Check sheet for the modelled part. Datum: model origin and axes. Units: mm. A direction names the side the tool comes from. Give positions to 0.01 mm unless a question says otherwise; leave off trailing zeros. Order: outer loops, then holes, each group sorted by start corner. A loop starts at its lowest first (then second) coordinate and runs counter-clockwise, first axis right, second up. Notation, with made-up numbers: M 52,67.5 L 72,67.5 A19 ccw 72,80.5 Z; hole C 9.5,22.5 d2. An arc over 180 degrees is marked long. Answer in a Markdown table with one row per item. Add a question column.
from build123d import *

# Parameters (mm, degrees)
SKETCH1_R           = 1.6500000000000001
SKETCH1_R_2         = 1.6500000000000006
BOSS_EXTRUDE1_DEPTH = 2
BOSS_EXTRUDE2_DEPTH = 2
BOSS_EXTRUDE3_DEPTH = 4
SKETCH4_R           = 1.8999999999999948
SKETCH4_R_2         = 1.8999999999999981
CUT_EXTRUDE1_DEPTH  = 4
SKETCH5_R           = 1.0000000000000009
SKETCH5_R_2         = 1
SKETCH5_R_3         = 1.8999999999999981
CUT_EXTRUDE2_DEPTH  = 63.418667079648536
CUT_EXTRUDE3_DEPTH  = 4
CHAMFER1_SIZE       = 5
CHAMFER2_SIZE       = 2
FILLET1_R           = 8
FILLET2_R           = 8
FILLET3_R           = 8


# Some blends are built 0.0001 mm under size
with BuildPart() as part:
    # Sketch1 → Boss-Extrude1 (new body)
    with BuildSketch(Plane.XY):
        Polygon((0, 0), (-12, -1.47e-15), (-12, 45), (0, 45), align=None)
        with Locations((-6.499999999999999, 37)):
            Circle(SKETCH1_R, mode=Mode.SUBTRACT)
        with Locations((-6.5000000000000036, 5.999999999999999)):
            Circle(SKETCH1_R_2, mode=Mode.SUBTRACT)
    extrude(amount=-BOSS_EXTRUDE1_DEPTH)

    # Sketch2 → Boss-Extrude2 (add)
    with BuildSketch(Plane(origin=(0, 0, 0), x_dir=(0, 0, -1), z_dir=(1, 0, 0))):
        Polygon((35.3, 45), (2, 0), (5.51e-15, 0), (0, 45), align=None)
    extrude(amount=BOSS_EXTRUDE2_DEPTH)

    # Sketch3 → Boss-Extrude3 (add)
    with BuildSketch(Plane(origin=(0, 45, 0), x_dir=(1, 0, 0), z_dir=(0, 1, 0))):
        Polygon((-6.1e-16, 35.3), (25, 35.3), (25.000000000000004, 1.9999999999999991), (3.47e-15, 1.9999999999999991), align=None)
    extrude(amount=-BOSS_EXTRUDE3_DEPTH)

    # Sketch4 → Cut-Extrude1 (cut)
    with BuildSketch(Plane(origin=(0, 45, 0), x_dir=(1, 0, 0), z_dir=(0, 1, 0))):
        with Locations(Location((20.000000000000004, 26.850000000000005, 0), (0, 0, 270))):
            Circle(SKETCH4_R)
        with Locations(Location((20.00000000000001, 16.45, 0), (0, 0, 270))):
            Circle(SKETCH4_R)
        with Locations(Location((11.200000000000008, 21.650000000000002, 0), (0, 0, 270))):
            Circle(SKETCH4_R_2)
    extrude(amount=-CUT_EXTRUDE1_DEPTH, mode=Mode.SUBTRACT)

    # Sketch5 → Cut-Extrude2 (cut, through all)
    with BuildSketch(Plane(origin=(0, 45, 0), x_dir=(1, 0, 0), z_dir=(0, 1, 0))):
        with Locations(Location((3.5826389249908894, 23.65, 0), (0, 0, 270))):
            Circle(SKETCH5_R)
        with Locations(Location((3.5826389249908894, 19.650000000000002, 0), (0, 0, 270))):
            Circle(SKETCH5_R_2)
        with Locations(Location((11.200000000000008, 21.650000000000002, 0), (0, 0, 270))):
            Circle(SKETCH5_R_3)
    extrude(amount=-CUT_EXTRUDE2_DEPTH, mode=Mode.SUBTRACT)

    # Sketch6 → Cut-Extrude3 (cut)
    with BuildSketch(Plane(origin=(0, 45, 0), x_dir=(1, 0, 0), z_dir=(0, 1, 0))):
        Polygon((13.000000000000005, 1.9999999999999991), (25.000000000000004, 13.999999999999877), (25.000000000000004, 1.9999999999999991), align=None)
    extrude(amount=-CUT_EXTRUDE3_DEPTH, mode=Mode.SUBTRACT)

    # Chamfer1
    # the kernel refuses this chamfer: 5 mm, written as the material it adds along each edge
    with BuildSketch(Plane(origin=(2, 41, -45.19841493982955), x_dir=(-0.02749587661058636, -0.9996219169112968, 0), z_dir=(0, 0, 1))) as chamfer1_piece_1_section:
        Polygon((CHAMFER1_SIZE * 0.999621916911, CHAMFER1_SIZE * 0.0274958766106), (-CHAMFER1_SIZE * 0.0274958766106, CHAMFER1_SIZE * 0.999621916911), (0, 0), align=None)
    chamfer1_piece_1 = extrude(amount=43.19841493982955, mode=Mode.PRIVATE)
    chamfer1_piece_1 = split(chamfer1_piece_1, bisect_by=Plane(origin=(3.679771833975431, 32.284665683470884, -25.89065260576845), z_dir=(0, 0.5948430054102947, 0.8038418992031009)), keep=Keep.TOP, mode=Mode.PRIVATE)
    chamfer1_piece_1 = chamfer1_piece_1 - Plane(origin=(3.5826389249908894, 39.396771086693036, -19.650000000000002), x_dir=(-1.8e-16, 0, 1), z_dir=(0, 1, 0)) * Cylinder(1, 107, mode=Mode.PRIVATE)
    chamfer1_piece_1 = chamfer1_piece_1 - Plane(origin=(3.5826389249908894, 39.396771086693036, -23.65), x_dir=(-1.8e-16, 0, 1), z_dir=(0, 1, 0)) * Cylinder(1.0000000000000009, 107, mode=Mode.PRIVATE)
    add(chamfer1_piece_1)

    # Chamfer2
    chamfer2_edges = [part.edges().sort_by_distance(p)[0] for p in [
        (1.9999999999990004, 40.50000000000074, -1.9999999999999996),
    ]]
    chamfer(chamfer2_edges, length=CHAMFER2_SIZE - 0.0001)  # a hair under: the kernel refuses the full size

    # Fillet1
    fillet1_edges = [part.edges().sort_by_distance(p)[0] for p in [
        (-12, -1.47e-15, -1),
        (-12, 45, -1),
    ]]
    fillet(fillet1_edges, radius=FILLET1_R)

    # Fillet2
    fillet2_edges = [part.edges().sort_by_distance(p)[0] for p in [
        (-6.1e-16, 43, -35.3),
        (25, 43, -35.3),
    ]]
    fillet(fillet2_edges, radius=FILLET2_R)

    # Fillet3
    fillet3_edges = [part.edges().sort_by_distance(p)[0] for p in [
        (13.000000000000005, 43, -1.9999999999999991),
        (25.000000000000004, 43, -13.999999999999877),
    ]]
    fillet(fillet3_edges, radius=FILLET3_R)


solid = part.part
Q1. Tool access check on faces 4 (the flat face through (6, 42, -2)), 5 (the flat face through (-1, 0, -1)), 6 (the flat face through (-6, 23, -2)). Record the directions out of +Z, -Z, +X, -X, +Y, -Y that give a thin tool (end or side, any length) a straight path to the whole face; none if there is none.
Q2. Thickness scan on probe 1 along Y at (x, z) = (-6.5, -0.45); probe 2 along X at (y, z) = (43, -23.65); probe 3 along Y at (x, z) = (14, -15.5). Record the ranges inside material, lowest first.
Q3. Cross-section at D-D (y = 29). Record the boundary of the cut face in (x, z), and give its area (3 significant figures).
Q4. Cross-section at A-A (x = 11.2). Record the boundary of the cut face in (y, z), and give its area (3 significant figures).
Q5. Cross-section at C-C (z = -28). Record the boundary of the cut face in (x, y), and give its area (3 significant figures).
Q6. Go/stop test with flat-tipped pins: pin 1 (1.5 mm diameter, centred on x = 13, z = -31.5, fed in from -Y); pin 2 (1 mm diameter, centred on x = -2, z = -28, fed in from +Y); pin 3 (12 mm diameter, centred on y = 33, z = -25, fed in from -X); pin 4 (4 mm diameter, centred on x = -6.5, y = 37, fed in from -Z). Record where each tip stops, or that it passes through.
Q7. Draft check along Z on faces 1 (the cylindrical face through (-7.716, 38.115, -0.986)), 2 (the flat face through (1.41, 21.92, -18.22)), 3 (the cylindrical face through (2.606, 40.804, -19.867)). Enter one of: pulls with the +Z half, pulls with the -Z half, needs draft (parallel to the pull), parting line crosses it, or undercut.
Q8. Cross-section at B-B (x = -6.5). Record the boundary of the cut face in (y, z), and give its area (3 significant figures).
Values follow:
| question | item | result |
|---|---|---|
| 1 | face 4 | +Z, +X, +Y, -Y |
| 1 | face 5 | +Z, -Z, +X, -X, -Y |
| 1 | face 6 | -Z, -X, +Y, -Y |
| 2 | probe 1 | 0.4 to 4.35, 7.65 to 35.35, 38.65 to 44.6 |
| 2 | probe 2 | 0 to 2.58, 4.58 to 25 |
| 2 | probe 3 | 41 to 45 |
| 3 | outline | M -12,-2 L 0,-2 L 0,-23.46 L 2,-23.46 L 2,0 L -12,0 Z |
| 3 | area | 70.9 mm² |
| 4 | outline | M 41,-35.3 L 45,-35.3 L 45,-23.55 L 41,-23.55 Z; M 41,-19.75 L 45,-19.75 L 45,-2.14 L 41,-2.14 Z |
| 4 | area | 117 mm² |
| 5 | outline | M 0.03,35.14 L 2,35.14 L 2,36 L 7,41 L 18.49,41 L 18.49,45 L 0.03,45 Z; M 21.51,41 L 24.97,41 L 24.97,45 L 21.51,45 Z |
| 5 | area | 112 mm² |
| 6 | pin 1 | y = 41 |
| 6 | pin 2 | through |
| 6 | pin 3 | x = 0 |
| 6 | pin 4 | z = -2 |
| 7 | face 1 | needs draft |
| 7 | face 2 | pulls with the -Z half |
| 7 | face 3 | undercut |
| 8 | outline | M 0.4,-2 L 4.35,-2 L 4.35,0 L 0.4,0 Z; M 7.65,-2 L 35.35,-2 L 35.35,0 L 7.65,0 Z; M 38.65,-2 L 44.6,-2 L 44.6,0 L 38.65,0 Z |
| 8 | area | 75.2 mm² |
